Geometry: final body of the model. Coordinates: model frame, mm. A direction names the side the tool comes from. Give positions to 0.01 mm unless a question says otherwise; leave off trailing zeros. Write each loop counter-clockwise with the first axis right and the second up, starting at its lowest first coordinate (ties: lowest second). Pieces come first, ordered by that corner, then holes.
Q1. Pin query (flat end, axial travel): pin 1 Ø3 at (y, z) = (31, 1.5) entering from +X; pin 2 Ø1 at (x, z) = (-56, 1.5) entering from -Y. Return the tip coordinate at first contact, or that it passes through.
Q2. Section C-C (y = 27). Return the cut outline in (x, z), plus the area to 3 significant figures.
Q3. Section B-B (x = 33). Return the cut outline in (y, z), plus the area to 3 significant figures.
Q4. Mould query, pull axis Y, two halves, no side actions, for faces 1 (the cylindrical face through (-54.74, 68.59, 3.22)), 2 (the flat face through (26.004, 136.831, 3.219)), 3 (the flat face through (-1, 33, 0)). Classes: +Y half, -Y half, draft (parallel to the pull), parting line (faces both ways), or undercut.
Q5. Line query: line 1 (Y direction, x = -25, z = 4); line 2 (Y direction, x = -38, z = 3.25); line 3 (X direction, y = 116, z = 0.75). Output: solid intervals per line, ascending.
Q6. Section A-A (z = 4.5). Return the cut outline in (x, y), plus the area to 3 significant figures.
Q7. Reachability of faces 4 (the flat face through (-56.6, 57.5, 3.2)), 5 (the flat face through (56.203, 58.016, 3.219)), 6 (the flat face through (-1, 33, 6.35)) from +Z, -Z, +X, -X, +Y, -Y: full face, straight path, thin tool, end or side. Return the list, or none.
from build123d import *

# Parameters (mm, degrees)
F1_DEPTH = 6.35
F2_R     = 12.7
F4_DEPTH = 6.351


# Not quite as in the source:
# - a feature names something its author has since deleted; it is built from what else it names


with BuildPart() as f1:
    # F0 (on Top) → F1 (new body)
    with BuildSketch(Plane.XY):
        with BuildLine():
            ThreePointArc((-70.543128599, 41.1726645916), (-70.7849997477, 40.4855010306), (-71.1039826136, 39.8305618399))
            ThreePointArc((-71.1039826136, 39.8305618399), (-1.0804242799, -81.4928382336), (72.1349447987, 37.9315137965))
            Line((72.1349447987, 37.9315137965), (64.1774671745, 49.691417374))
            Line((64.1774671745, 49.691417374), (60.7204563849, 68.6290463558))
            ThreePointArc((60.7204563849, 68.6290463558), (58.8124253174, 109.8022050591), (31.9532798351, 141.0664959374))
            Line((31.9532798352, 141.0664959374), (24.5, 144.5356458426))
            Line((24.5, 144.5356458426), (0, 144.5356458426))
            Line((0, 144.5356458426), (-24.5, 144.5356458426))
            Line((-24.5, 144.5356458426), (-31.9532798352, 141.0664959374))
            ThreePointArc((-31.9532798351, 141.0664959374), (-58.8010464391, 109.8308374249), (-60.7377773112, 68.688183064))
            Line((-60.7377773112, 68.688183064), (-64.7292534015, 49.691417374))
            Line((-64.7292534015, 49.691417374), (-70.543128599, 41.1726645916))
        make_face()
    extrude(amount=F1_DEPTH)

    # F2
    f2_edges = [f1.edges().sort_by_distance(p)[0] for p in [
        (60.720456, 68.629046, 3.175),
        (72.134945, 37.931514, 3.175),
        (64.177467, 49.691417, 3.175),
        (-64.729253, 49.691417, 3.175),
        (-60.737777, 68.688183, 3.175),
    ]]
    fillet(f2_edges, radius=F2_R)

    # F3 (on face) → F4 (cut, through all)
    with BuildSketch(Plane.XY.offset(6.35)):
        with BuildLine():
            ThreePointArc((-70.543128599, 41.1726645916), (-70.7849997477, 40.4855010306), (-71.1039826136, 39.8305618399))
            ThreePointArc((-71.1039826136, 39.8305618399), (-1.4798729053, -81.4865631634), (72.5033392644, 37.2225173183))
            ThreePointArc((72.5033392644, 37.2225173183), (72.133296657, 37.8927702646), (71.7235387193, 38.5395074414))
            Line((71.7235387193, 38.5395074414), (65.673391241, 47.4806762809))
            ThreePointArc((65.673391241, 47.4806762809), (64.4343566454, 49.7963304465), (63.6981152819, 52.3173242185))
            Line((63.6981152819, 52.3173242185), (61.235654247, 65.8067740057))
            ThreePointArc((61.235654247, 65.8067740057), (61.0355921512, 68.4904493527), (61.4054899639, 71.1560288055))
            ThreePointArc((61.4054899639, 71.1560288055), (58.3166642414, 111.0138701005), (31.9532798351, 141.0664959374))
            Line((31.9532798352, 141.0664959374), (24.5, 144.5356458426))
            Line((24.5, 144.5356458426), (-24.5, 144.5356458426))
            Line((-24.5, 144.5356458426), (-31.9532798352, 141.0664959374))
            ThreePointArc((-31.9532798351, 141.0664959374), (-58.2757571875, 111.1107457801), (-61.4559677961, 71.3601980865))
            ThreePointArc((-61.4559677961, 71.3601980865), (-61.0915979292, 68.5460068659), (-61.3611887293, 65.7211602459))
            Line((-61.3611887293, 65.7211602459), (-64.2110715476, 52.1576176071))
            ThreePointArc((-64.2110715476, 52.1576176071), (-64.9570302406, 49.7885224974), (-66.149830538, 47.6099235298))
            Line((-66.149830538, 47.6099235298), (-70.543128599, 41.1726645916))
        make_face()
        with BuildLine():
            Line((-28.9966635349, 135.438502816), (-23.0945782645, 138.1856448808))
            Line((-23.0945782645, 138.1856448808), (23.0945782645, 138.1856448808))
            Line((23.0945782645, 138.1856448808), (28.9966635349, 135.438502816))
            ThreePointArc((28.9966635349, 135.438502816), (52.520857183, 108.4149325541), (55.243636, 72.6903260202))
            ThreePointArc((55.243636, 72.6903260202), (54.6887892531, 68.6919566393), (54.988882412, 64.6664434155))
            Line((54.988882412, 64.6664434155), (57.4513434469, 51.1769936283))
            ThreePointArc((57.4513434469, 51.1769936283), (58.5557055478, 47.3955027794), (60.4142575351, 43.9220213556))
            Line((60.4142575351, 43.9220213556), (66.4644050134, 34.9808525161))
            ThreePointArc((66.4644050134, 34.9808525161), (66.6692839512, 34.6574839767), (66.8543052269, 34.3223575543))
            ThreePointArc((66.8543052269, 34.3223575543), (-1.3645699068, -75.137609121), (-65.5639782212, 36.7271985762))
            ThreePointArc((-65.5639782212, 36.7271985762), (-65.1678300151, 37.4944518277), (-64.8247337429, 38.2868506548))
            Line((-64.8247337429, 38.2868506548), (-60.904901379, 44.0303662485))
            ThreePointArc((-60.904901379, 44.0303662485), (-59.1157008425, 47.2982648647), (-57.9967627465, 50.8519077088))
            Line((-57.9967627465, 50.8519077088), (-55.1468799282, 64.4154503476))
            ThreePointArc((-55.1468799282, 64.4154503476), (-54.7424937077, 68.6527204915), (-55.2890485355, 72.8740075355))
            ThreePointArc((-55.2890485355, 72.8740075355), (-52.4842770002, 108.5021804525), (-28.9966635349, 135.438502816))
        make_face(mode=Mode.SUBTRACT)
    extrude(amount=-F4_DEPTH, mode=Mode.SUBTRACT)


solid = f1.part
Computed:
1. pin 1: stops at x = 69.12
1. pin 2: stops at y = -50.67
2. outline: (-70.13, 0) - (70.13, 0) - (70.13, 6.35) - (-70.13, 6.35) - close
2. area: 891 mm2
3. outline: (-67.52, 0) - (132.84, 0) - (132.84, 6.35) - (-67.52, 6.35) - close
3. area: 1,270 mm2
4. face 1: undercut
4. face 2: +Y half
4. face 3: draft
5. line 1: y = -70.87 to 137.3
5. line 2: y = -64.83 to 128.84
5. line 3: x = -48.66 to 48.66
6. outline: (-65.56, 36.73) arc R75.15 ccw (long way) to (66.85, 34.32) arc R6.35 ccw to (66.46, 34.98) - (60.41, 43.92) arc R19.05 cw to (57.45, 51.18) - (54.99, 64.67) arc R19.05 cw to (55.24, 72.69) arc R56.93 ccw to (29, 135.44) - (23.09, 138.19) - (-23.09, 138.19) - (-29, 135.44) arc R56.93 ccw to (-55.29, 72.87) arc R19.05 cw to (-55.15, 64.42) - (-58, 50.85) arc R19.05 cw to (-60.9, 44.03) - (-64.82, 38.29) arc R12.7 cw to start
6. area: 24,800 mm2
7. face 4: +Z, -Z, -X
7. face 5: +Z, -Z, +X
7. face 6: +Z, +X, -X, +Y, -Y
